Autodesk Inventor part; units mm, degrees
ref_plane "YZ Plane" through (0, 0, 0) normal (1, 0, 0) x (0, 1, 0)
ref_plane "XZ Plane" through (0, 0, 0) normal (0, 1, 0) x (-1, 0, 0)
ref_plane "XY Plane" through (0, 0, 0) normal (0, 0, 1) x (1, 0, 0)
sketch "スケッチ1" plane through (0, 0, 0) normal (0, 0, 1) x (1, 0, 0)
  line L0 (-170.6512, -31.4118) -> (202.8656, -31.4118) construction
  circle A0 centre (-14, -17.4118) radius 14 construction
  circle A1 centre (14, -17.4118) radius 14 construction
  circle A2 centre (-28.0204, 0.0121) radius 20.05 construction
  circle A3 centre (-28.0204, 0.0121) radius 5.05 construction
  circle A4 centre (8.8763, 3.8907) radius 32.05 construction
  circle A5 centre (8.8763, 3.8907) radius 10.1 construction
  circle A6 centre (54.047, 13.5882) radius 36.1 construction
  line L1 (-170.915, -81.4118) -> (490.0044, -81.4118)
  circle A7 centre (-28.0204, 0.0121) radius 22.342 construction
  circle A8 centre (-39.4931, 19.1835) radius 14 construction
  circle A9 centre (-49.0547, 7.5438) radius 14 construction
  circle A10 centre (-49.0547, -7.5196) radius 14 construction
  circle A11 centre (-39.4931, -19.1593) radius 14 construction
  circle A12 centre (8.8763, 3.8907) radius 33.05 construction
  circle A13 centre (54.047, 13.5882) radius 38.1 construction
  line L2 (-11.5565, -29.1593) -> (4.2969, -29.1593) construction
  line L3 (-67.2952, 44.8622) -> (-67.2952, -57.3934) construction
  line L4 (-149.4523, -1.6098) -> (-132.6633, -31.6026)
  line L5 (-132.7701, -31.4118) -> (-132.7701, 74.0456)
  circle A14 centre (-11.4931, -19.1593) radius 14 construction
  line L6 (-197.2268, -33.1593) -> (179.6604, -33.1593) construction
  circle A15 centre (54.047, 13.5882) radius 4.025 construction
  circle A16 centre (54.047, 13.5882) radius 6 construction
  circle A17 centre (-39.4931, 19.1835) radius 5
  circle A18 centre (-49.0547, 7.5438) radius 5
  circle A19 centre (-49.0547, -7.5196) radius 5
  circle A20 centre (-39.4931, -19.1593) radius 5
  circle A21 centre (-39.4931, 19.1835) radius 8 construction
  circle A22 centre (-49.0547, 7.5438) radius 8 construction
  circle A23 centre (-49.0547, -7.5196) radius 8 construction
  circle A24 centre (-39.4931, -19.1593) radius 8 construction
  circle A25 centre (-28.0204, 0.0121) radius 4.5
  circle A26 centre (8.8763, 3.8907) radius 7.5
  line L7 (-17.5497, 32.3149) -> (-46.3578, 15.0755) construction
  line L8 (-46.3578, 15.0755) -> (-51.7515, 0.0121) construction
  line L9 (-51.7515, 0.0121) -> (-46.3578, -15.0513) construction
  line L10 (-46.3578, -15.0513) -> (-37.9391, -20.0892) construction
  circle A27 centre (-32.6283, 23.2915) radius 1.3
  circle A28 centre (-46.3578, 15.0755) radius 1.3
  circle A29 centre (-51.7515, 0.0121) radius 1.3
  circle A30 centre (-46.3578, -15.0513) radius 1.3
  circle A31 centre (-32.6283, -23.2673) radius 1.3
  line L11 (-67.2952, 23.1796) -> (-67.2952, -18.1327)
  arc A32 (79.2003, -37.212) -> (87.3507, -31.2711) centre (80.4159, -30.3183) ccw
  arc A33 (8.1864, 50.8943) -> (0.9804, 51.9708) centre (3.7003, 45.5208) ccw
  line L12 (-52.2685, -33.1593) -> (56.2168, -33.1593)
  line L13 (56.2168, -33.1593) -> (79.2003, -37.212)
  arc A34 (92.7831, 8.2659) -> (29.742, 44.2162) centre (54.047, 13.5882) ccw
  line L14 (87.3507, -31.2711) -> (92.7831, 8.2659)
  line L15 (0.9804, 51.9708) -> (-67.2952, 23.1796)
  circle A35 centre (34.0114, -24.0061) radius 4.5 construction
  circle A36 centre (34.0114, -24.0061) radius 1.5
  circle A37 centre (-21.4477, 26.0369) radius 4.5 construction
  circle A38 centre (-21.4477, 26.0369) radius 1.5
  circle A39 centre (-56.0504, 23.0377) radius 1.5
  circle A40 centre (-56.0504, 23.0377) radius 3 construction
  circle A41 centre (-56.0504, 23.0377) radius 4.5 construction
  circle A42 centre (-64.2952, 0.0121) radius 1.5
  circle A43 centre (-64.2952, 0.0121) radius 3 construction
  circle A44 centre (-64.2952, 0.0121) radius 4.3311 construction
  line L16 (54.047, 13.5882) -> (99.37, -7.5264)
  line L17 (99.37, -7.5264) -> (58.3399, 10.9541)
  line L18 (58.3399, 10.9541) -> (30.7326, 32.4678)
  line L19 (30.7326, 32.4678) -> (54.047, 13.5882)
  line L20 (99.37, -7.5264) -> (491.4359, -184.1173)
  line L21 (-183.2789, 162.2213) -> (-183.2789, -125.2315)
  line L22 (516.7211, 155.5913) -> (516.7211, -155.5644)
  circle A45 centre (99.37, -7.5264) radius 7.25
  line L23 (149.518, -30.1136) -> (397.5027, -198.9436) construction
  line L24 (220.2014, -78.2354) -> (225.3858, -8.4277) construction
  circle A46 centre (3.7003, 45.5208) radius 4
  circle A47 centre (135.8413, -23.9534) radius 2
  circle A48 centre (149.518, -30.1136) radius 2
  arc A49 (147.9092, -34.8477) -> (151.9972, -25.7715) centre (149.518, -30.1136) ccw
  line L25 (147.9092, -34.8477) -> (96.0719, -17.2312)
  line L26 (151.9972, -25.7715) -> (104.4523, 1.3749)
  circle A50 centre (30.7326, 32.4678) radius 2
  circle A51 centre (-16.1798, -24.0771) radius 4.5 construction
  circle A52 centre (-16.1798, -24.0771) radius 1.5
  line L27 (-67.2952, -18.1327) -> (-52.2685, -33.1593)
  circle A53 centre (-56.0504, -23.0135) radius 1.5
  circle A54 centre (-56.0504, -23.0135) radius 3 construction
  circle A55 centre (30.7326, 32.4678) radius 4
  arc A56 (56.8403, 15.6972) -> (51.3644, 11.3402) centre (54.047, 13.5882) ccw construction
  line L28 (96.4916, -6.1854) -> (101.9705, -5.7041) construction
  line L29 (101.9705, -5.7041) -> (99.6479, -10.6896) construction
  line L30 (99.6479, -10.6896) -> (96.4916, -6.1854) construction
  circle A57 centre (99.6479, -10.6896) radius 1.5
  circle A58 centre (101.9705, -5.7041) radius 1.5
  circle A59 centre (96.4916, -6.1854) radius 1.5
  circle A60 centre (99.37, -7.5264) radius 6
  arc A61 (97.7876, -15.8778) -> (97.5111, 0.7679) centre (99.37, -7.5264) ccw
  arc A62 (56.8403, 15.6972) -> (97.5111, 0.7679) centre (88.7632, 39.7996) ccw
  arc A63 (51.3644, 11.3402) -> (97.7876, -15.8778) centre (112.6811, 62.7237) ccw
  circle A64 centre (54.047, 13.5882) radius 8.5 construction
  line L31 (102.9595, 0.1786) -> (57.6365, 21.2931) construction
  line L32 (50.4575, 5.8833) -> (95.7806, -15.2313) construction
  circle A65 centre (12.7384, 41.2415) radius 3 construction
  circle A66 centre (12.7384, 41.2415) radius 4.5 construction
  circle A67 centre (12.7384, 41.2415) radius 1.5
  circle A68 centre (80.4159, -30.3183) radius 4
  circle A69 centre (69.7531, -26.0108) radius 1.5
  circle A70 centre (69.7531, -26.0108) radius 4.5 construction
  circle A71 centre (-56.0504, -23.0135) radius 4.5 construction
  line L33 (8.1864, 50.8943) -> (15.9809, 44.3871)
  arc A72 (15.9809, 44.3871) -> (29.742, 44.2162) centre (22.9664, 52.7545) ccw
  circle A73 centre (-5.4761, 38.5895) radius 1.5
  circle A74 centre (-5.4761, 38.5895) radius 4.5 construction
  circle A75 centre (54.047, 13.5882) radius 50 construction
  circle A76 centre (3.7003, 45.5208) radius 2
  circle A77 centre (80.4159, -30.3183) radius 2
  circle A78 centre (54.047, 13.5882) radius 1.5
  circle A79 centre (58.3399, 10.9541) radius 1.5
  circle A80 centre (58.3399, 10.9541) radius 3
  arc A81 (59.8474, 15.7214) -> (55.7687, 6.6659) centre (58.3399, 10.9541) ccw
  line L34 (94.099, -16.3172) -> (55.7687, 6.6659)
  line L35 (59.8474, 15.7214) -> (102.4604, 2.2467)
  arc A82 (104.4523, 1.3749) -> (102.4604, 2.2467) centre (99.37, -7.5264) ccw
  arc A83 (94.099, -16.3172) -> (96.0719, -17.2312) centre (99.37, -7.5264) ccw
  circle A84 centre (30.7326, 32.4678) radius 5.025
  circle A85 centre (30.7326, 32.4678) radius 8.025
  circle A86 centre (58.3399, 10.9541) radius 4.025
  circle A87 centre (58.3399, 10.9541) radius 7.025
  line L36 (25.9827, 25.9995) -> (54.1819, 5.2918)
  line L37 (53.3095, 15.8577) -> (37.1861, 27.6978)
  line L38 (65.3516, 11.3852) -> (66.2721, -3.5865)
  line L39 (66.2721, -3.5865) -> (54.1819, 5.2918)
  line L40 (67.2722, 8.2659) -> (69.0337, -1.2879)
  line L41 (67.2722, 8.2659) -> (82.8858, 8.4364)
  point P0 (0, 0)
  point P1 (0, 0)
  point P2 (0, 0)
  point P3 (-49.0547, 7.5438)
  point P4 (-49.0547, -7.5196)
  dimension "d88" = 100
  dimension "d0" = 40.1
  dimension "d1" = 10.1
  dimension "d2" = 64.1
  dimension "d3" = 20.2
  dimension "d4" = 72.2
  dimension "d5" = 95
  dimension "d6" = 44.684
  dimension "d7" = 28
  dimension "d8" = 28
  dimension "d9" = 28
  dimension "d10" = 28
  dimension "d11" = 1
  dimension "d12" = 2
  dimension "d13" = 4
  dimension "d14" = 8.05
  dimension "d15" = 12
  dimension "d16" = 10
  dimension "d17" = 10
  dimension "d18" = 10
  dimension "d19" = 10
  dimension "d20" = 3
  dimension "d21" = 3
  dimension "d22" = 3
  dimension "d23" = 3
  dimension "d24" = 9
  dimension "d25" = 15
  dimension "d26" = 2.6
  dimension "d27" = 2.6
  dimension "d28" = 2.6
  dimension "d29" = 2.6
  dimension "d30" = 2.6
  dimension "d31" = 1
  dimension "d32" = 9
  dimension "d33" = 3
  dimension "d34" = 9
  dimension "d35" = 3
  dimension "d36" = 3
  dimension "d37" = 6
  dimension "d38" = 9
  dimension "d39" = 3
  dimension "d40" = 6
  dimension "d41" = 50
  dimension "d42" = 45
  dimension "d43" = 35
  dimension "d44" = 30
  dimension "d45" = 39
  dimension "d46" = 430
  dimension "d47" = 700
  dimension "d48" = 14.5
  dimension "d49" = 300
  dimension "d50" = 10
  dimension "d51" = 70
  dimension "d52" = 120
  dimension "d53" = 140
  dimension "d54" = 8
  dimension "d55" = 4
  dimension "d56" = 4
  dimension "d57" = 15
  dimension "d58" = 40
  dimension "d59" = 10
  dimension "d60" = 4
  dimension "d61" = 9
  dimension "d62" = 3
  dimension "d63" = 3
sketch "スケッチ2" plane through (0, 0, 0) normal (0, 0, 1) x (1, 0, 0)
  circle A0 centre (149.518, -30.1136) radius 2
  circle A1 centre (135.8413, -23.9534) radius 2
  line L0 (151.9972, -25.7715) -> (104.4523, 1.3749)
  arc A2 (147.9092, -34.8477) -> (151.9972, -25.7715) centre (149.518, -30.1136) ccw
  line L1 (147.9092, -34.8477) -> (96.0719, -17.2312)
  circle A3 centre (142.6796, -27.0335) radius 1.65
  circle A4 centre (156.3563, -33.1937) radius 1.65
  line L2 (135.8413, -23.9534) -> (213.3942, -58.8842)
  circle A5 centre (142.6796, -27.0335) radius 5 construction
  circle A6 centre (150.426, -41.4901) radius 1.25
  arc A7 (147.3765, -44.4504) -> (153.4081, -44.5182) centre (150.426, -41.4901) ccw
  line L3 (154.5328, -32.3723) -> (140.4569, -63.6234) construction
  line L4 (154.3028, -43.2363) -> (188.3811, -58.5855) construction
  line L5 (160.5664, -37.4686) -> (153.4081, -44.5182)
  arc A8 (138.3053, -18.4827) -> (131.5361, -28.1326) centre (135.8413, -23.9534) ccw
  line L6 (158.8204, -27.723) -> (138.3053, -18.4827)
  line L7 (147.3765, -44.4504) -> (131.5361, -28.1326)
  arc A9 (160.5664, -37.4686) -> (158.8204, -27.723) centre (156.3563, -33.1937) ccw
  point P0 (0, 0)
  dimension "d104" = 3.3
  dimension "d105" = 3.3
  dimension "d106" = 15
  dimension "d107" = 10
  dimension "d109" = 2.5
  dimension "d110" = 3
  dimension "d111" = 13
  dimension "d112" = 10
  dimension "d113" = 6
  dimension "d114" = 6
  dimension "d115" = 7.5
extrude "押し出し1" add sketch "スケッチ2" along normal blind 18 contours A2 L1 L7 A8 L6 L0 | A2 L0 L6 A9 L2 A4 | L2 A4 A9 L5 A7 L7 L1 A2
sketch "スケッチ3" plane through (0, 0, 18) normal (0, 0, 1) x (1, 0, 0)
  circle A0 centre (135.8413, -23.9534) radius 2
  circle A1 centre (149.518, -30.1136) radius 2
  circle A2 centre (156.3563, -33.1937) radius 1.65
  circle A3 centre (142.6796, -27.0335) radius 1.65
  circle A4 centre (150.426, -41.4901) radius 1.25
  line L0 (153.4081, -44.5182) -> (160.5664, -37.4686)
  arc A5 (160.5664, -37.4686) -> (158.8204, -27.723) centre (156.3563, -33.1937) ccw
  line L1 (158.8204, -27.723) -> (138.3053, -18.4827)
  arc A6 (138.3053, -18.4827) -> (131.5361, -28.1326) centre (135.8413, -23.9534) ccw
  line L2 (131.5361, -28.1326) -> (147.3765, -44.4504)
  arc A7 (147.3765, -44.4504) -> (153.4081, -44.5182) centre (150.426, -41.4901) ccw
  circle A8 centre (135.8413, -23.9534) radius 4
  circle A9 centre (149.518, -30.1136) radius 4
  point P0 (0, 0)
  dimension "d118" = 8
  dimension "d119" = 8
extrude "押し出し2" cut sketch "スケッチ3" against normal blind 12 contours A8 | A9
extrude "押し出し3" cut sketch "スケッチ1" along normal blind 3 contours L35 A82 L26 A49 L20 A48 A47 A61 A62 L14 | L14 A62 L16 L40 L41 L35 | L34 L40 A62 L17 L14 | L14 L17 A45 L20 A61 A63 L34 | A63 A61 L20 A47 A48 A49 L25 A83 L34 | A62 A61 L20 A45 L16 L14 | L14 L16 A62 | L17 A62 L16 L14 | L14 L16 A45 L17 | A62 L17 L40 L16 | A62 L40 L17
properties part number "アダプター" material "アルミニウム 7075"
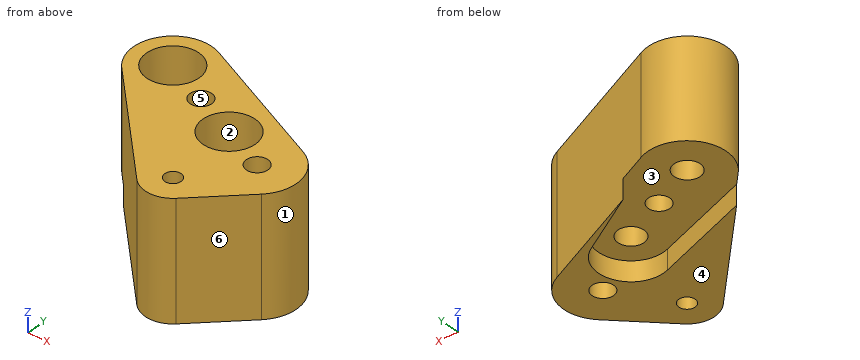
The model under review builds one solid part; all positions refer to its coordinate system, in mm. Face numbers are marked on the shaded views. A direction names the side the tool comes from. Coordinates: 2 decimals unless noted, no trailing zeros. Loops run counter-clockwise (first coordinate to the right, second up) from the corner with the lowest first, then second, coordinate; pieces in that order, holes last. Notation, with made-up numbers: (4, 7.25) -> (26, 7.25) arc R19 cw to (26, 15.25) -> close; hole circle Ø7 at (21, 55.5). An arc over 180 degrees is marked (long way). Use a Markdown table: item, result. Add a question column.
1. Clearance check with flat-ended pins moving along their axes: pin 1 Ø1.5 at (x, z) = (147.5, 3.5) entering from +Y; pin 2 Ø1.5 at (x, z) = (143.5, 3) entering from -Y; pin 3 Ø10.5 at (x, y) = (135.84, -23.95) entering from -Z. State where each tip first meets the part, or that it passes through.
2. Draft analysis for pull direction Y (two halves, no side actions). For the marked faces 4, 5 and 6, state which applies: pulls with the +Y half, pulls with the -Y half, needs draft (parallel to the pull), parting line crosses it, or undercut.
3. Add section C-C on x = 151. Write out the cut boundary in (y, z).
4. Add section A-A on x = 136. Write out the cut boundary in (y, z), plus the area to 3 significant figures.
5. To check wall thickness, follow line 1 (X direction, y = -33.5, z = 10.25); line 2 (Y direction, x = 151, z = 15.5); line 3 (Y direction, x = 155.5, z = 9). State the ranges of each line that lie inside material, in increasing order.
6. Add section D-D on y = -25. Write out the cut boundary in (x, z), plus the area to 3 significant figures.
7. Machinability: for the marked faces 1, 2 and 3, which of the approach directions +Z, -Z, +X, -X, +Y, -Y give a long, thin tool a straight path to every point of the face, cutting with its end or side? Answer none if there is none.
8. Add section B-B on z = 6.5. Write out the cut boundary in (x, y).
Returned:
| question | item | result |
|---|---|---|
| 1 | pin 1 | stops at y = -22.29 |
| 1 | pin 2 | stops at y = -41.23 |
| 1 | pin 3 | stops at z = 3 |
| 2 | face 4 | needs draft |
| 2 | face 5 | undercut |
| 2 | face 6 | pulls with the -Y half |
| 3 | outline | (-45.7, 0) -> (-42.6, 0) -> (-42.6, 18) -> (-45.7, 18) -> close; (-40.38, 0) -> (-34.89, 0) -> (-34.89, 3) -> (-31.46, 3) -> (-31.46, 6) -> (-33.83, 6) -> (-33.83, 18) -> (-40.38, 18) -> close; (-28.77, 3) -> (-25.2, 3) -> (-25.2, 0) -> (-24.2, 0) -> (-24.2, 18) -> (-26.4, 18) -> (-26.4, 6) -> (-28.77, 6) -> close |
| 4 | outline | (-32.73, 0) -> (-30.8, 0) -> (-30.8, 3) -> (-25.95, 3) -> (-25.95, 6) -> (-27.95, 6) -> (-27.95, 18) -> (-32.73, 18) -> close; (-21.96, 3) -> (-17.96, 3) -> (-17.96, 18) -> (-19.96, 18) -> (-19.96, 6) -> (-21.96, 6) -> close |
| 4 | area | 120 mm² |
| 5 | line 1 | x = 136.75 to 147.39, 151.65 to 154.73, 157.98 to 162.35 |
| 5 | line 2 | y = -45.7 to -42.6, -40.38 to -33.83, -26.4 to -24.2 |
| 5 | line 3 | y = -42.46 to -34.6, -31.78 to -26.23 |
| 6 | outline | (129.93, 3) -> (134.14, 3) -> (134.14, 6) -> (131.98, 6) -> (131.98, 18) -> (129.93, 18) -> close; (137.55, 3) -> (150.65, 3) -> (150.65, 0) -> (152.77, 0) -> (152.77, 18) -> (139.7, 18) -> (139.7, 6) -> (137.55, 6) -> close |
| 6 | area | 246 mm² |
| 7 | face 1 | +Z, -Z, +X |
| 7 | face 2 | +Z |
| 7 | face 3 | -Z |
| 8 | outline | (131.54, -28.13) -> (147.38, -44.45) arc R4.25 ccw to (153.41, -44.52) -> (160.57, -37.47) arc R6 ccw to (158.82, -27.72) -> (138.31, -18.48) arc R6 ccw to start; hole circle Ø8 at (135.84, -23.95); hole circle Ø3.3 at (142.68, -27.03); hole circle Ø8 at (149.52, -30.11); hole circle Ø2.5 at (150.43, -41.49); hole circle Ø3.3 at (156.36, -33.19) |
